from build123d import *

# Parameters (mm, degrees)
BOX_W             = 130
BOX_H             = 73
BOX_DEPTH         = 2
BOX001_W          = 35
BOX001_H          = 49
BOX001_DEPTH      = 4
CYLINDER_R        = 17.5
CYLINDER_DEPTH    = 14
BOX002_W          = 63
BOX002_H          = 51
BOX002_DEPTH      = 3
CYLINDER001_R     = 17.5
CYLINDER001_DEPTH = 10
CYLINDER002_R     = 1.5
CYLINDER002_DEPTH = 3
CYLINDER003_R     = 1.5
CYLINDER003_DEPTH = 3
CYLINDER004_R     = 1.5
CYLINDER004_DEPTH = 3
CYLINDER005_R     = 1.5
CYLINDER005_DEPTH = 3
CYLINDER006_R     = 1.5
CYLINDER006_DEPTH = 3
CYLINDER007_R     = 1.5
CYLINDER007_DEPTH = 3
BOX003_W          = 2
BOX003_H          = 10
BOX003_DEPTH      = 3
BOX004_W          = 5
BOX004_H          = 5
BOX004_DEPTH      = 3
CYLINDER008_R     = 1.25
CYLINDER008_DEPTH = 2
CYLINDER009_R     = 1.25
CYLINDER009_DEPTH = 2
CYLINDER010_R     = 1.25
CYLINDER010_DEPTH = 2
CYLINDER011_R     = 1.25
CYLINDER011_DEPTH = 2
FILLET_R          = 1.5
FILLET001_R       = 1.5
FILLET002_R       = 1.5
FILLET003_R       = 1.5


with BuildPart() as part:
    # Box → Box (join)
    with BuildSketch(Plane.XY):
        with Locations((65, 36.5)):
            Rectangle(BOX_W, BOX_H)
    extrude(amount=BOX_DEPTH)

    # Box001 → Box001 (cut)
    with BuildSketch(Plane(origin=(13, 12.5, -2), x_dir=(1, 0, 0), z_dir=(0, 0, 1))):
        with Locations((17.5, 24.5)):
            Rectangle(BOX001_W, BOX001_H)
    extrude(amount=BOX001_DEPTH, mode=Mode.SUBTRACT)

    # Cylinder → Cylinder (cut)
    with BuildSketch(Plane(origin=(90, 40.5, -6), x_dir=(1, 0, 0), z_dir=(0, 0, 1))):
        Circle(CYLINDER_R)
    extrude(amount=CYLINDER_DEPTH, mode=Mode.SUBTRACT)

    # Box002 → Box002 (join)
    with BuildSketch(Plane(origin=(65, 21, -3), x_dir=(1, 0, 0), z_dir=(0, 0, 1))):
        with Locations((31.5, 25.5)):
            Rectangle(BOX002_W, BOX002_H)
    extrude(amount=BOX002_DEPTH)

    # Cylinder001 → Cylinder001 (cut)
    with BuildSketch(Plane(origin=(90, 40.5, -5), x_dir=(1, 0, 0), z_dir=(0, 0, 1))):
        Circle(CYLINDER001_R)
    extrude(amount=CYLINDER001_DEPTH, mode=Mode.SUBTRACT)

    # Cylinder002 → Cylinder002 (cut)
    with BuildSketch(Plane(origin=(106, 24.5, 0), x_dir=(1, 0, 0), z_dir=(0, 0, -1))):
        Circle(CYLINDER002_R)
    extrude(amount=CYLINDER002_DEPTH, mode=Mode.SUBTRACT)

    # Cylinder003 → Cylinder003 (cut)
    with BuildSketch(Plane(origin=(74, 24.5, 0), x_dir=(1, 0, 0), z_dir=(0, 0, -1))):
        Circle(CYLINDER003_R)
    extrude(amount=CYLINDER003_DEPTH, mode=Mode.SUBTRACT)

    # Cylinder004 → Cylinder004 (cut)
    with BuildSketch(Plane(origin=(74, 56.5, 0), x_dir=(1, 0, 0), z_dir=(0, 0, -1))):
        Circle(CYLINDER004_R)
    extrude(amount=CYLINDER004_DEPTH, mode=Mode.SUBTRACT)

    # Cylinder005 → Cylinder005 (cut)
    with BuildSketch(Plane(origin=(106, 56.5, 0), x_dir=(1, 0, 0), z_dir=(0, 0, -1))):
        Circle(CYLINDER005_R)
    extrude(amount=CYLINDER005_DEPTH, mode=Mode.SUBTRACT)

    # Cylinder006 → Cylinder006 (cut)
    with BuildSketch(Plane(origin=(116.5, 41.5, 0), x_dir=(1, 0, 0), z_dir=(0, 0, -1))):
        Circle(CYLINDER006_R)
    extrude(amount=CYLINDER006_DEPTH, mode=Mode.SUBTRACT)

    # Cylinder007 → Cylinder007 (cut)
    with BuildSketch(Plane(origin=(116.5, 31.5, 0), x_dir=(1, 0, 0), z_dir=(0, 0, -1))):
        Circle(CYLINDER007_R)
    extrude(amount=CYLINDER007_DEPTH, mode=Mode.SUBTRACT)

    # Box003 → Box003 (join)
    with BuildSketch(Plane(origin=(128, 41.5, 0), x_dir=(1, 0, 0), z_dir=(0, 0, -1))):
        with Locations((1, 5)):
            Rectangle(BOX003_W, BOX003_H)
    extrude(amount=BOX003_DEPTH)

    # Box004 → Box004 (cut)
    with BuildSketch(Plane(origin=(123, 67, -3), x_dir=(1, 0, 0), z_dir=(0, 0, 1))):
        with Locations((2.5, 2.5)):
            Rectangle(BOX004_W, BOX004_H)
    extrude(amount=BOX004_DEPTH, mode=Mode.SUBTRACT)

    # Cylinder008 → Cylinder008 (cut)
    with BuildSketch(Plane(origin=(3, 69.5, 0), x_dir=(1, 0, 0), z_dir=(0, 0, 1))):
        Circle(CYLINDER008_R)
    extrude(amount=CYLINDER008_DEPTH, mode=Mode.SUBTRACT)

    # Cylinder009 → Cylinder009 (cut)
    with BuildSketch(Plane(origin=(3, 3.5, 0), x_dir=(1, 0, 0), z_dir=(0, 0, 1))):
        Circle(CYLINDER009_R)
    extrude(amount=CYLINDER009_DEPTH, mode=Mode.SUBTRACT)

    # Cylinder010 → Cylinder010 (cut)
    with BuildSketch(Plane(origin=(126.5, 3.5, 0), x_dir=(1, 0, 0), z_dir=(0, 0, 1))):
        Circle(CYLINDER010_R)
    extrude(amount=CYLINDER010_DEPTH, mode=Mode.SUBTRACT)

    # Cylinder011 → Cylinder011 (cut)
    with BuildSketch(Plane(origin=(126.5, 69.5, 0), x_dir=(1, 0, 0), z_dir=(0, 0, 1))):
        Circle(CYLINDER011_R)
    extrude(amount=CYLINDER011_DEPTH, mode=Mode.SUBTRACT)

    # Fillet
    fillet_edges = [part.edges().sort_by_distance(p)[0] for p in [
        (65, 0, 2),
    ]]
    fillet(fillet_edges, radius=FILLET_R)

    # Fillet001
    fillet001_edges = [part.edges().sort_by_distance(p)[0] for p in [
        (130, 37.25, 2),
    ]]
    fillet(fillet001_edges, radius=FILLET001_R)

    # Fillet002
    fillet002_edges = [part.edges().sort_by_distance(p)[0] for p in [
        (64.25, 73, 2),
    ]]
    fillet(fillet002_edges, radius=FILLET002_R)

    # Fillet003
    fillet003_edges = [part.edges().sort_by_distance(p)[0] for p in [
        (0, 36.5, 2),
    ]]
    fillet(fillet003_edges, radius=FILLET003_R)


solid = part.part
Geometry check sheet. Reference: the model listing, model coordinates, mm. A direction names the side the tool comes from. Give positions to 0.01 mm unless a question says otherwise; leave off trailing zeros. Loops run counter-clockwise (first coordinate to the right, second up) from the corner with the lowest first, then second, coordinate; pieces in that order, holes last. Notation, with made-up numbers: M 47,-7 L 57,-7 A9 cw 57,2 Z; hole C 55,-9.5 d7. An arc over 180 degrees is marked long. Answer as a JSON object with one key per item and string values. Group by question number.
Item 1: Material ranges on L1, parallel to Y at x = 116.5, z = -1.9; L2, parallel to Y at x = 3, z = 0.9; L3, parallel to X at y = 43, z = 1.6, recorded low to high.
Item 2: Mould release check, pull along X, two halves, no side actions. Record for faces 5 (the flat face through (96, 21, -2)), 6 (the cylindrical face through (75.43, 56.05, -1.48)), 7 (the flat face through (123, 69, -2)), 8 (the cylindrical face through (127.69, 69.88, 0.99)): pulls with the +X half, pulls with the -X half, needs draft (parallel to the pull), parting line crosses it, or undercut.
Item 3: Sectioned sample at C-C on x = 28.5. Record the boundary of the cut face in (y, z), plus the area to 3 significant figures.
Item 4: Gauge pin test, flat ends, axial feed: pin 1 (3.5 mm diameter, centred on x = 74, y = 24.5, fed in from -Z); pin 2 (0.9 mm diameter, centred on x = 116.5, y = 31, fed in from -Z); pin 3 (1.5 mm diameter, centred on y = 30, z = -2, fed in from +X); pin 4 (0.9 mm diameter, centred on x = 82, z = -1.5, fed in from -Y). Record the tip position at first contact, or that the pin passes through.
Item 5: Sectioned sample at A-A on x = 3. Record the boundary of the cut face in (y, z), plus the area to 3 significant figures.
Item 6: Access from +Z, -Z, +X, -X, +Y, -Y to the whole of each face (thin tool, end or side, straight path). Record for faces 1 (the flat face through (128, 54, -2)), 2 (the flat face through (128, 26, -2)), 3 (the flat face through (65, 46, -2)), 4 (the cylindrical face through (104.89, 55.49, -1.48)).
Item 7: Sectioned sample at B-B on y = 38.5. Record the boundary of the cut face in (x, z).
Item 8: Sectioned sample at D-D on y = 7.5. Record the boundary of the cut face in (x, z), plus the area to 3 significant figures.
Findings below:
{
 "1": {"L1": "21 to 30, 33 to 40, 43 to 72", "L2": "0.05 to 2.25, 4.75 to 68.25, 70.75 to 72.95", "L3": "0.48 to 13, 48 to 72.68, 107.32 to 129.52"},
 "2": {"face 5": "needs draft", "face 6": "undercut", "face 7": "pulls with the +X half", "face 8": "undercut"},
 "3": {"outline": "M 0,0 L 12.5,0 L 12.5,2 L 1.5,2 A1.5 ccw 0,0.5 Z; M 61.5,0 L 73,0 L 73,0.5 A1.5 ccw 71.5,2 L 61.5,2 Z", "area": "47.0 mm2"},
 "4": {"pin 1": "z = -3", "pin 2": "z = 0", "pin 3": "x = 128", "pin 4": "y = 21"},
 "5": {"outline": "M 0,0 L 2.25,0 L 2.25,2 L 1.5,2 A1.5 ccw 0,0.5 Z; M 4.75,0 L 68.25,0 L 68.25,2 L 4.75,2 Z; M 70.75,0 L 73,0 L 73,0.5 A1.5 ccw 71.5,2 L 70.75,2 Z", "area": "135 mm2"},
 "6": {"face 1": "-Z, +X, +Y", "face 2": "-Z, +X, -Y", "face 3": "-Z, -X, +Y, -Y", "face 4": "-Z"},
 "7": {"outline": "M 0,0 L 13,0 L 13,2 L 1.5,2 A1.5 ccw 0,0.5 Z; M 48,0 L 65,0 L 65,-3 L 72.61,-3 L 72.61,2 L 48,2 Z; M 107.39,-3 L 130,-3 L 130,0.5 A1.5 ccw 128.5,2 L 107.39,2 Z"},
 "8": {"outline": "M 0,0 L 130,0 L 130,0.5 A1.5 ccw 128.5,2 L 1.5,2 A1.5 ccw 0,0.5 Z", "area": "259 mm2"}
}
